```python
from build123d import *

# Parameters (mm, degrees)
BOSS_EXTRUDE1_DEPTH = 22
SKETCH2_W           = 32.324702558
SKETCH2_H           = 10
CUT_EXTRUDE1_DEPTH  = 22
FILLET2_R           = 2


with BuildPart() as part:
    # Sketch1 → Boss-Extrude1 (new body)
    with BuildSketch(Plane.XY):
        Polygon((-2.531920895, 4.378113215), (-7.546246883, 6.382242673), (-6.989544256, 7.775111003), (-2.24326139, 5.878113215), (52.413753117, 5.878113215), (52.413753117, 4.378113215), align=None)
    extrude(amount=BOSS_EXTRUDE1_DEPTH)

    # Sketch2 → Cut-Extrude1 (cut)
    with BuildSketch(Plane.XZ.offset(-4.378113215)):
        with Locations((1.251401838, 17)):
            Rectangle(SKETCH2_W, SKETCH2_H)
        with BuildLine():
            Line((28.876886466, 15), (28.876886466, 5))
            ThreePointArc((28.876886466, 5), (27.413753117, 3.536866651), (25.950619767, 5))
            Line((25.950619767, 5), (25.950619767, 15))
            ThreePointArc((25.950619767, 15), (27.413753117, 16.463133349), (28.876886466, 15))
        make_face()
        with BuildLine():
            Line((43.757050896, 15), (43.757050896, 5))
            ThreePointArc((43.757050896, 5), (42.413753117, 3.656702221), (41.070455337, 5))
            Line((41.070455337, 5), (41.070455337, 15))
            ThreePointArc((41.070455337, 15), (42.413753117, 16.343297779), (43.757050896, 15))
        make_face()
    extrude(amount=-CUT_EXTRUDE1_DEPTH, mode=Mode.SUBTRACT)

    # Fillet2
    fillet2_edges = [part.edges().sort_by_distance(p)[0] for p in [
        (17.413753117, 5.128113215, 22),
        (-7.26789557, 7.078676838, 12),
        (17.413753117, 5.128113215, 12),
        (-7.26789557, 7.078676838, 0),
    ]]
    fillet(fillet2_edges, radius=FILLET2_R)


solid = part.part
```
Input: part model. Units: mm. Frame: model coordinates. A direction names the side the tool comes from. Coordinates: 2 decimals unless noted, no trailing zeros. Write each loop counter-clockwise with the first axis right and the second up, starting at its lowest first coordinate (ties: lowest second). Pieces come first, ordered by that corner, then holes. Notation, with made-up numbers: M 57,67.5 L 101,67.5 A19 cw 101,103.5 Z; hole C 38.5,62.25 d9. An arc over 180 degrees is marked long. Use one line per item in the form item = value.
Q1. Set-up query: faces 1 (the face through (43.757, 5, 10)), 2 (the face through (5, 5, 12)), 3 (the face through (25, 5.878, 11)). Return all of +Z, -Z, +X, -X, +Y, -Y with unobstructed straight access to the full face (end or side cutting, diameter ignored); none if empty.
Answer below:
face_1 = +Y, -Y
face_2 = +Z, -X, +Y, -Y
face_3 = +Z, -Z, +X, +Y
Q2. Material intervals for probe 1 along X at (y, z) = (5.15, 14.25); probe 2 along X at (y, z) = (4.8, 15.5); probe 3 along Y at (x, z) = (17.5, 11), sorted ascending. Write a range as from..to.
Answer below:
probe_1 = 17.41..25.95, 28.88..41.07, 43.76..52.41
probe_2 = 17.41..26.04, 28.79..41.17, 43.66..52.41
probe_3 = 4.38..5.88
Q3. Section D-D (x = 12). Return loops of the section in (y, z), plus the area to 3 significant figures.
Answer below:
outline = M 4.38,0 L 5.88,0 L 5.88,12 L 4.38,12 Z
area = 18.0 mm²
Q4. Section A-A (z = 8.5). Return loops of the section in (x, y), plus the area to 3 significant figures.
Answer below:
outline = M -7.55,6.38 L -2.53,4.38 L 25.95,4.38 L 25.95,5.88 L -2.24,5.88 L -6.99,7.78 Z; M 28.88,4.38 L 41.07,4.38 L 41.07,5.88 L 28.88,5.88 Z; M 43.76,4.38 L 52.41,4.38 L 52.41,5.88 L 43.76,5.88 Z
area = 81.7 mm²
Q5. Section B-B (x = 43). Return loops of the section in (y, z).
Answer below:
outline = M 4.38,0 L 5.88,0 L 5.88,3.79 L 4.38,3.79 Z; M 4.38,16.21 L 5.88,16.21 L 5.88,22 L 4.38,22 Z
Q6. First-contact query: pin 1 (0.8 mm diameter, centred on y = 5, z = 17.5, fed in from -X); pin 2 (6 mm diameter, centred on x = 40, z = 10, fed in from +Y); pin 3 (0.8 mm diameter, centred on x = 9.5, y = 5, fed in from +Z). Flat tips, straight axial feed; report the tip coordinate or a pass-through.
Answer below:
pin_1 = 17.41
pin_2 = 5.88
pin_3 = 12
Q7. Section C-C (y = 4.9). Return loops of the section in (x, z), plus the area to 3 significant figures.
Answer below:
outline = M -3.84,0 L 52.41,0 L 52.41,22 L 19.41,22 A2 ccw 17.41,20 L 17.41,14 A2 cw 15.41,12 L -3.84,12 Z; hole M 25.95,5 A1.46 ccw 28.88,5 L 28.88,15 A1.46 ccw 25.95,15 Z; hole M 41.07,5 A1.34 ccw 43.76,5 L 43.76,15 A1.34 ccw 41.07,15 Z
area = 956 mm²
